Could you check a few things on this model? Use its own coordinates, in mm. Face numbers are marked on the shaded views. A direction names the side the tool comes from. Coordinates: 2 decimals unless noted, no trailing zeros. Loops run counter-clockwise (first coordinate to the right, second up) from the corner with the lowest first, then second, coordinate; pieces in that order, holes last. Notation, with made-up numbers: (12.5, 46.5) -> (39.5, 46.5) arc R32 ccw to (39.5, 80.5) -> close; hole circle Ø1 at (53.25, 89.25). An arc over 180 degrees is marked (long way). One line per question, with ' | ' between items.
from build123d import *

# Parameters (mm, degrees)
SKETCH1_W           = 140
SKETCH1_H           = 200
SKETCH1_R           = 7.5
BOSS_EXTRUDE1_DEPTH = 10
SKETCH2_W           = 5
SKETCH2_H           = 200
BOSS_EXTRUDE2_DEPTH = 25
SKETCH3_R           = 5
CUT_EXTRUDE1_DEPTH  = 176.570498661
SKETCH4_R           = 45
SKETCH4_R_2         = 35
BOSS_EXTRUDE3_DEPTH = 70
FILLET1_R           = 10


with BuildPart() as part:
    # Sketch1 → Boss-Extrude1 (new body)
    with BuildSketch(Plane.XY):
        Rectangle(SKETCH1_W, SKETCH1_H)
        with Locations((-50, -50)):
            Circle(SKETCH1_R, mode=Mode.SUBTRACT)
        with Locations((50, -50)):
            Circle(SKETCH1_R, mode=Mode.SUBTRACT)
    extrude(amount=BOSS_EXTRUDE1_DEPTH)

    # Sketch2 → Boss-Extrude2 (add)
    with BuildSketch(Plane.XY.offset(10)):
        with Locations((-67.5, 0)):
            Rectangle(SKETCH2_W, SKETCH2_H)
        with Locations((67.5, 0)):
            Rectangle(SKETCH2_W, SKETCH2_H)
    extrude(amount=BOSS_EXTRUDE2_DEPTH)

    # Sketch3 → Cut-Extrude1 (cut, through all)
    with BuildSketch(Plane.ZY.offset(70)):
        with Locations(Location((17.5, 85, 0), (0, 0, 270))):
            Circle(SKETCH3_R)
    extrude(amount=-CUT_EXTRUDE1_DEPTH, mode=Mode.SUBTRACT)

    # Sketch4 → Boss-Extrude3 (add)
    with BuildSketch(Plane(origin=(0, 0, 0), x_dir=(-1, 0, 0), z_dir=(0, 0, -1))):
        with Locations(Location((0, 0, 0), (0, 0, 180))):
            Circle(SKETCH4_R)
        Circle(SKETCH4_R_2, mode=Mode.SUBTRACT)
    extrude(amount=BOSS_EXTRUDE3_DEPTH)

    # Fillet1
    fillet1_edges = [part.edges().sort_by_distance(p)[0] for p in [
        (-45, 0, 0),
    ]]
    fillet(fillet1_edges, radius=FILLET1_R)


solid = part.part
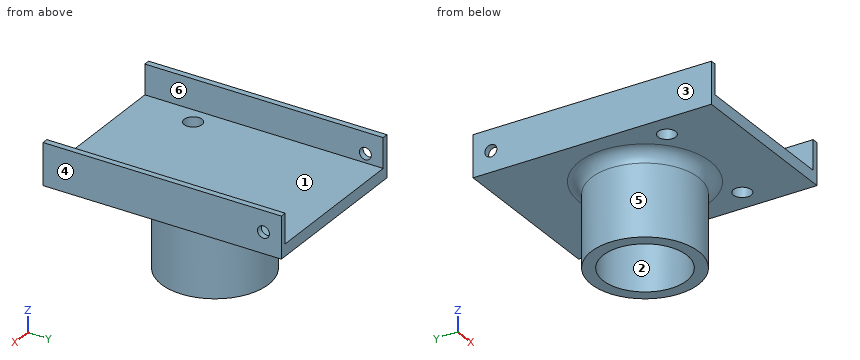
1) I need wall thicknesses on line 1 along X through (y, z) = (14, 21); line 2 along Y through (x, z) = (50, 7.5); line 3 along Y through (x, z) = (0, -18). Which ranges of each line are inside material? Lowest first, please. Write a range as from..to.
Data:
line 1: -70..-65, 65..70 | line 2: -100..-57.5, -42.5..100 | line 3: -45..-35, 35..45
2) If we section it at A-A on y = 85: Please give me the cut outline in (x, z), and give its area (3 significant figures).
Data:
outline: (-70, 0) -> (70, 0) -> (70, 12.5) -> (65, 12.5) -> (65, 10) -> (-65, 10) -> (-65, 12.5) -> (-70, 12.5) -> close; (-70, 22.5) -> (-65, 22.5) -> (-65, 35) -> (-70, 35) -> close; (65, 22.5) -> (70, 22.5) -> (70, 35) -> (65, 35) -> close | area: 1,550 mm²
3) If we section it at C-C on y = 0: Please give me the cut outline in (x, z), and give its area (3 significant figures).
Data:
outline: (-70, 0) -> (-55, 0) arc R10 cw to (-45, -10) -> (-45, -70) -> (-35, -70) -> (-35, 0) -> (35, 0) -> (35, -70) -> (45, -70) -> (45, -10) arc R10 cw to (55, 0) -> (70, 0) -> (70, 35) -> (65, 35) -> (65, 10) -> (-65, 10) -> (-65, 35) -> (-70, 35) -> close | area: 3,090 mm²
4) If we section it at D-D on z = -14.5: Please give me the cut outline in (x, y), and give its area (3 significant figures).
Data:
outline: circle Ø90 at (0, 0); hole circle Ø70 at (0, 0) | area: 2,510 mm²
5) I'm going to push flat-ended pins straight in: pin 1 Ø10 at (x, z) = (-47, -3.5) entering from +Y; pin 2 Ø1.5 at (y, z) = (-41, -45) entering from -X; pin 3 Ø12 at (x, y) = (50, -50) entering from -Z; pin 4 Ø12 at (x, y) = (6.5, 34.5) entering from +Z. Where does each tip first touch, or does it pass through?
Data:
pin 1: y = 100 | pin 2: x = -20.12 | pin 3: through | pin 4: z = 10
6) If we section it at B-B on z = 17.5: Please give me the cut outline in (x, y).
Data:
outline: (-70, -100) -> (-65, -100) -> (-65, 80) -> (-70, 80) -> close; (-70, 90) -> (-65, 90) -> (-65, 100) -> (-70, 100) -> close; (65, -100) -> (70, -100) -> (70, 80) -> (65, 80) -> close; (65, 90) -> (70, 90) -> (70, 100) -> (65, 100) -> close
7) We'd pull the mould along X, two halves only. Please class the marked faces 4, 5 and 6: pulls with the +X half, pulls with the -X half, needs draft (parallel to the pull), parting line crosses it, or undercut.
Data:
face 4: pulls with the +X half | face 5: parting line crosses it | face 6: undercut
8) On a 3-axis mill with a long thin cutter (end or side, diameter ignored), from which of +Z, -Z, +X, -X, +Y, -Y can I reach the whole of each face in a straight line? I mean the marked faces 1, 2 and 3. Say none if no direction works.
Data:
face 1: +Z, +Y, -Y | face 2: -Z | face 3: +Z, -Z, -X, +Y, -Y
